Read the model definition and answer for the solid it produces. Units are mm, in the model's axes. Face numbers are marked on the shaded views. A direction names the side the tool comes from. Coordinates: 2 decimals unless noted, no trailing zeros. Write each loop counter-clockwise with the first axis right and the second up, starting at its lowest first coordinate (ties: lowest second). Pieces come first, ordered by that corner, then holes. Notation, with made-up numbers: M -9.75,2 L 14.25,2 A22 cw 14.25,13 Z; hole C 3,-16 d7. An arc over 180 degrees is marked long. Use a Markdown table: item, result. Add a question column.
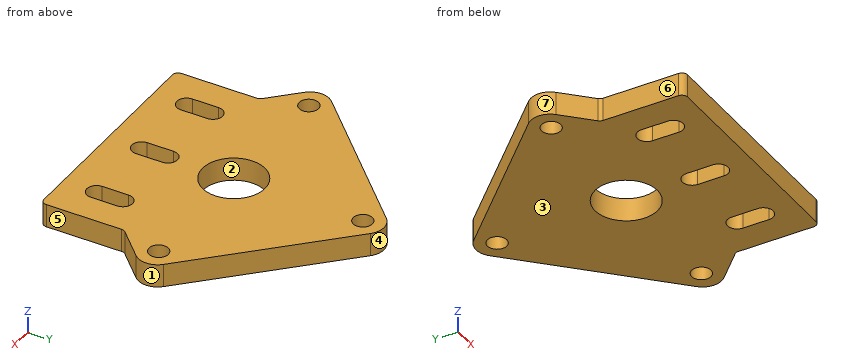
from build123d import *

# Parameters (mm, degrees)
F0_R     = 4.6
F0_R_2   = 8.05
F0_R_3   = 2.5
F1_DEPTH = 6


# Not quite as in the source:
# - ends of sketch curves that miss each other by under 0.0002 mm in the source are joined


with BuildPart() as f1:
    # F0 (on Top) → F1 (new body)
    with BuildSketch(Plane.XY):
        with BuildLine():
            ThreePointArc((-30, -34.104246), (-29.5606601718, -35.1649061718), (-28.5, -35.604246))
            Line((-28.5, -35.604246), (28.5, -35.604246))
            ThreePointArc((28.5, -35.604246), (29.5606601718, -35.1649061718), (30, -34.104246))
            Line((30, -34.104246), (30, -14.645125))
            ThreePointArc((30, -14.645125), (30.1141807012, -14.0710998515), (30.4393398282, -13.5844648282))
            Line((30.4393398282, -13.5844648282), (37.314025, -6.70978))
            ThreePointArc((37.314025, -6.70978), (38.778491, -3.174246), (37.3140249059, 0.3612879059))
            Line((37.3140249059, 0.3612879059), (3.535534, 34.139779))
            ThreePointArc((3.535534, 34.139779), (0, 35.604245), (-3.5355339059, 34.1397789059))
            Line((-3.5355339059, 34.1397789059), (-37.314025, 0.361288))
            ThreePointArc((-37.314025, 0.361288), (-38.778491, -3.174246), (-37.3140249059, -6.7097799059))
            Line((-37.3140249059, -6.7097799059), (-30.43934, -13.584465))
            ThreePointArc((-30.43934, -13.584465), (-30.1141807012, -14.0710998515), (-30, -14.645125))
            Line((-30, -14.645125), (-30, -34.104246))
        make_face()
        with BuildLine():
            ThreePointArc((-24.6, -20.174246), (-20, -15.574246), (-15.4, -20.174246))
            Line((-15.4, -20.174246), (-15.4, -26.974246))
            ThreePointArc((-15.4, -26.974246), (-20, -31.574246), (-24.6, -26.974246))
            Line((-24.6, -26.974246), (-24.6, -20.174246))
        make_face(mode=Mode.SUBTRACT)
        with Locations((-33.333, -3.174246)):
            Circle(F0_R, mode=Mode.SUBTRACT)
        with BuildLine():
            ThreePointArc((4.6, -26.974246), (0, -31.574246), (-4.6, -26.974246))
            Line((-4.6, -26.974246), (-4.6, -20.174246))
            ThreePointArc((-4.6, -20.174246), (0, -15.574246), (4.6, -20.174246))
            Line((4.6, -20.174246), (4.6, -26.974246))
        make_face(mode=Mode.SUBTRACT)
        with BuildLine():
            ThreePointArc((24.6, -26.974246), (20, -31.574246), (15.4, -26.974246))
            Line((15.4, -26.974246), (15.4, -20.174246))
            ThreePointArc((15.4, -20.174246), (20, -15.574246), (24.6, -20.174246))
            Line((24.6, -20.174246), (24.6, -26.974246))
        make_face(mode=Mode.SUBTRACT)
        with Locations((0, -3.174246)):
            Circle(F0_R_2, mode=Mode.SUBTRACT)
        with Locations((33.333, -3.174246)):
            Circle(F0_R, mode=Mode.SUBTRACT)
        with Locations((0, 30.158782)):
            Circle(F0_R, mode=Mode.SUBTRACT)
        with Locations((-33.333, -3.174246)):
            Circle(F0_R)
        with Locations((-33.333, -3.174246)):
            Circle(F0_R_3, mode=Mode.SUBTRACT)
        with Locations((0, 30.158782)):
            Circle(F0_R)
        with Locations((0, 30.158782)):
            Circle(F0_R_3, mode=Mode.SUBTRACT)
        with Locations((33.333, -3.174246)):
            Circle(F0_R)
        with Locations((33.333, -3.174246)):
            Circle(F0_R_3, mode=Mode.SUBTRACT)
        with BuildLine():
            Line((15.4, -20.174246), (15.4, -26.974246))
            ThreePointArc((15.4, -26.974246), (20, -31.574246), (24.6, -26.974246))
            Line((24.6, -26.974246), (24.6, -20.174246))
            ThreePointArc((24.6, -20.174246), (20, -15.574246), (15.4, -20.174246))
        make_face()
        with BuildLine():
            ThreePointArc((22.5, -26.974246), (20, -29.474246), (17.5, -26.974246))
            Line((17.5, -26.974246), (17.5, -20.174246))
            ThreePointArc((17.5, -20.174246), (20, -17.674246), (22.5, -20.174246))
            Line((22.5, -20.174246), (22.5, -26.974246))
        make_face(mode=Mode.SUBTRACT)
        with BuildLine():
            Line((-4.6, -20.174246), (-4.6, -26.974246))
            ThreePointArc((-4.6, -26.974246), (0, -31.574246), (4.6, -26.974246))
            Line((4.6, -26.974246), (4.6, -20.174246))
            ThreePointArc((4.6, -20.174246), (0, -15.574246), (-4.6, -20.174246))
        make_face()
        with BuildLine():
            ThreePointArc((2.5, -26.974246), (0, -29.474246), (-2.5, -26.974246))
            Line((-2.5, -26.974246), (-2.5, -20.174246))
            ThreePointArc((-2.5, -20.174246), (0, -17.674246), (2.5, -20.174246))
            Line((2.5, -20.174246), (2.5, -26.974246))
        make_face(mode=Mode.SUBTRACT)
        with BuildLine():
            Line((-15.4, -26.974246), (-15.4, -20.174246))
            ThreePointArc((-15.4, -20.174246), (-20, -15.574246), (-24.6, -20.174246))
            Line((-24.6, -20.174246), (-24.6, -26.974246))
            ThreePointArc((-24.6, -26.974246), (-20, -31.574246), (-15.4, -26.974246))
        make_face()
        with BuildLine():
            ThreePointArc((-17.5, -26.974246), (-20, -29.474246), (-22.5, -26.974246))
            Line((-22.5, -26.974246), (-22.5, -20.174246))
            ThreePointArc((-22.5, -20.174246), (-20, -17.674246), (-17.5, -20.174246))
            Line((-17.5, -20.174246), (-17.5, -26.974246))
        make_face(mode=Mode.SUBTRACT)
    extrude(amount=F1_DEPTH)


solid = f1.part
Item 1: Each of these flat-tipped pins is pushed along its axis until it touches: pin 1 (1 mm diameter, centred on x = -7, z = 5, fed in from +Y); pin 2 (3 mm diameter, centred on y = -19.5, z = 0.5, fed in from +X); pin 3 (1.5 mm diameter, centred on y = 21.5, z = 5.5, fed in from +X). Where does it stop, or does it pass through?
Item 2: Determine the mould class of the marked faces 1, 2, 3 and 4 for opening direction Y: pulls with the +Y half, pulls with the -Y half, needs draft (parallel to the pull), parting line crosses it, or undercut.
Item 3: Find section D-D on y = -10. Give the vertices of the cut face in (x, z), then the cut area to 3 significant figures.
Item 4: For the marked faces 5, 6 and 7, determine the directions among +Z, -Z, +X, -X, +Y, -Y from which every point of the face is accessible in a straight line to the end or side of a thin tool.
Item 5: Find section B-B on y = -21.5. Give the vertices of the cut face in (x, z), then the cut area to 3 significant figures.
Item 6: Find section A-A on x = 0. Give the vertices of the cut face in (y, z).
Item 7: Consider probe 1 along Y at (x, z) = (0, 2.35); probe 2 along X at (y, z) = (-25, 1.3); probe 3 along Y at (x, z) = (1, 1.95). Determine where each line is inside the solid, lowest interval first.
Item 8: Find section C-C on x = 20. Give the vertices of the cut face in (y, z), then the cut area to 3 significant figures.
Geometry says:
| question | item | result |
|---|---|---|
| 1 | pin 1 | stops at y = 31.18 |
| 1 | pin 2 | stops at x = 30 |
| 1 | pin 3 | stops at x = 16.93 |
| 2 | face 1 | parting line crosses it |
| 2 | face 2 | undercut |
| 2 | face 3 | needs draft |
| 2 | face 4 | pulls with the +Y half |
| 3 | outline | M -34.02,0 L -4.27,0 L -4.27,6 L -34.02,6 Z; M 4.27,0 L 34.02,0 L 34.02,6 L 4.27,6 Z |
| 3 | area | 357 mm2 |
| 4 | face 5 | +Z, -Z, +X, -Y |
| 4 | face 6 | +Z, -Z, -X, -Y |
| 4 | face 7 | +Z, -Z, -X |
| 5 | outline | M -30,0 L -22.5,0 L -22.5,6 L -30,6 Z; M -17.5,0 L -2.5,0 L -2.5,6 L -17.5,6 Z; M 2.5,0 L 17.5,0 L 17.5,6 L 2.5,6 Z; M 22.5,0 L 30,0 L 30,6 L 22.5,6 Z |
| 5 | area | 270 mm2 |
| 6 | outline | M -35.6,0 L -29.47,0 L -29.47,6 L -35.6,6 Z; M -17.67,0 L -11.22,0 L -11.22,6 L -17.67,6 Z; M 4.88,0 L 27.66,0 L 27.66,6 L 4.88,6 Z; M 32.66,0 L 35.6,0 L 35.6,6 L 32.66,6 Z |
| 7 | probe 1 | y = -35.6 to -29.47, -17.67 to -11.22, 4.88 to 27.66, 32.66 to 35.6 |
| 7 | probe 2 | x = -30 to -22.5, -17.5 to -2.5, 2.5 to 17.5, 22.5 to 30 |
| 7 | probe 3 | y = -35.6 to -29.27, -17.88 to -11.16, 4.81 to 27.87, 32.45 to 35.5 |
| 8 | outline | M -35.6,0 L -29.47,0 L -29.47,6 L -35.6,6 Z; M -17.67,0 L 17.68,0 L 17.68,6 L -17.67,6 Z |
| 8 | area | 249 mm2 |
